Source: CAD feature listing. Evaluate the final solid. Frame: model axes, mm. Face numbers are marked on the shaded views. A direction names the side the tool comes from. Round coordinates to 2 decimals unless told otherwise and drop trailing zeros. Order: outer loops, then holes, each group sorted by start corner. A loop starts at its lowest first (then second) coordinate and runs counter-clockwise, first axis right, second up. Notation, with made-up numbers: (-9.5, 88) -> (10.5, 88) arc R22 cw to (10.5, 111) -> close; hole circle Ø10 at (47.5, -16.75). An arc over 180 degrees is marked (long way). Write item = value, one per line. Start each with the question number.
(1) Cut plane C-C on z = 5. Return the cut outline in (x, y) (3 decimals), then the cut area to 3 significant figures.
(2) Draft query along Y for the marked faces 3, 4 and 5. Return one class per face: released by +Y, released by -Y, zero draft, split by the parting line, or undercut.
(3) Reachability of the marked faces 1 and 2 from +Z, -Z, +X, -X, +Y, -Y: full face, straight path, thin tool, end or side. Return the list, or none.
(4) Cut plane D-D on y = 5.25. Return the cut outline in (x, z), then the cut area to 3 significant figures.
(5) Cut plane B-B on x = 40.5. Return the cut outline in (y, z), then the cut area to 3 significant figures.
(6) Ray query, line 1 (X direction, y = 9.2, z = 0) (3 decimals); line 2 (X direction, y = 9.85, z = 5) (3 decimals); line 3 (Y direction, x = -9, z = 5.5). Return the intervals inside material, ascending.
(7) Cut plane A-A on x = 26. Return the cut outline in (y, z) (3 decimals).
(8) Contact query for a flat-ended pin moving along its axis: pin 1 Ø2.5 at (x, z) = (26, 5) entering from -Y. Output: stop coordinate, or through.
from build123d import *

# Parameters (mm, degrees)
SKETCH_1_W          = 20
SKETCH_1_H          = 20
SKETCH_1_W_2        = 18
SKETCH_1_H_2        = 18
EXTRUDE_1_DEPTH     = 50
SKETCH_2_R          = 2.025
SKETCH_2_R_2        = 3.025
CUT_EXTRUDE_1_DEPTH = 40


with BuildPart() as part:
    # 草图1 → 凸台-拉伸1 (new body, symmetric)
    with BuildSketch(Plane(origin=(0, 0, 0), x_dir=(0, 0, -1), z_dir=(1, 0, 0))):
        Rectangle(SKETCH_1_W, SKETCH_1_H)
        Rectangle(SKETCH_1_W_2, SKETCH_1_H_2, mode=Mode.SUBTRACT)
    extrude(amount=EXTRUDE_1_DEPTH, both=True)

    # 草图2 → 切除-拉伸1 (cut)
    with BuildSketch(Plane(origin=(0, 10, 0), x_dir=(1, 0, 0), z_dir=(0, 1, 0))):
        with Locations((26, 5)):
            Circle(SKETCH_2_R)
        with Locations((46, 5)):
            Circle(SKETCH_2_R)
        with Locations((46, -5)):
            Circle(SKETCH_2_R)
        with Locations((26, -5)):
            Circle(SKETCH_2_R)
        with Locations((36, 0)):
            Circle(SKETCH_2_R_2)
        with Locations((-45, 0)):
            Circle(SKETCH_2_R)
        with Locations((-25, 0)):
            Circle(SKETCH_2_R)
        with Locations((-35, 0)):
            Circle(SKETCH_2_R_2)
    extrude(amount=-CUT_EXTRUDE_1_DEPTH, mode=Mode.SUBTRACT)


solid = part.part
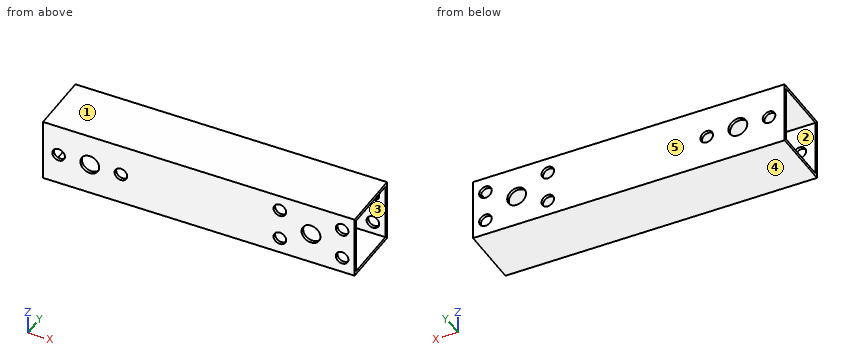
Evaluation:
q1.outline = (-50, -10) -> (23.975, -10) -> (23.975, -9) -> (-50, -9) -> close; (-50, 9) -> (23.975, 9) -> (23.975, 10) -> (-50, 10) -> close; (28.025, -10) -> (43.975, -10) -> (43.975, -9) -> (28.025, -9) -> close; (28.025, 9) -> (43.975, 9) -> (43.975, 10) -> (28.025, 10) -> close; (48.025, -10) -> (50, -10) -> (50, -9) -> (48.025, -9) -> close; (48.025, 9) -> (50, 9) -> (50, 10) -> (48.025, 10) -> close
q1.area = 184 mm^2
q2.face_3 = undercut
q2.face_4 = zero draft
q2.face_5 = released by +Y
q3.face_1 = +Z, +X, -X, +Y, -Y
q3.face_2 = +X, -X
q4.outline = (-50, -10) -> (50, -10) -> (50, -9) -> (-50, -9) -> close; (-50, 9) -> (50, 9) -> (50, 10) -> (-50, 10) -> close
q4.area = 200 mm^2
q5.outline = (-10, -10) -> (10, -10) -> (10, 10) -> (-10, 10) -> close; hole (-9, -9) -> (9, -9) -> (9, 9) -> (-9, 9) -> close
q5.area = 76.0 mm^2
q6.line_1 = -50 to -47.025, -42.975 to -38.025, -31.975 to -27.025, -22.975 to 32.975, 39.025 to 50
q6.line_2 = -50 to 23.975, 28.025 to 43.975, 48.025 to 50
q6.line_3 = -10 to -9, 9 to 10
q7.outline = (-10, -10) -> (10, -10) -> (10, -7.025) -> (9, -7.025) -> (9, -9) -> (-9, -9) -> (-9, -7.025) -> (-10, -7.025) -> close; (-10, -2.975) -> (-9, -2.975) -> (-9, 2.975) -> (-10, 2.975) -> close; (-10, 7.025) -> (-9, 7.025) -> (-9, 9) -> (9, 9) -> (9, 7.025) -> (10, 7.025) -> (10, 10) -> (-10, 10) -> close; (9, -2.975) -> (10, -2.975) -> (10, 2.975) -> (9, 2.975) -> close
q8.pin_1 = through
